```python
from build123d import *

# Parameters (mm, degrees)
SALIENTE_EXTRUIR1_DEPTH = 14
CROQUIS3_R              = 1.75
CORTAR_EXTRUIR1_DEPTH   = 30
REDONDEO3_R             = 4
REDONDEO4_R             = 2


with BuildPart() as part:
    # Croquis2 → Saliente-Extruir1 (new, symmetric)
    with BuildSketch(Plane(origin=(0, 0, 0), x_dir=(0, 0, -1), z_dir=(1, 0, 0))):
        with BuildLine():
            Line((-3, 1.5), (8, 1.5))
            Line((8, 1.5), (8, -1.5))
            Line((8, -1.5), (-8, -1.5))
            Line((-8, -1.5), (-8, 1.5))
            Line((-8, 1.5), (-8, 13.5))
            Line((-8, 13.5), (-5, 13.5))
            Line((-5, 13.5), (-5, 3.5))
            ThreePointArc((-5, 3.5), (-4.414213562, 2.085786438), (-3, 1.5))
        make_face()
    extrude(amount=SALIENTE_EXTRUIR1_DEPTH, both=True)

    # Croquis3 → Cortar-Extruir1 (cut)
    with BuildSketch(Plane(origin=(0, 1.5, 0), x_dir=(1, 0, 0), z_dir=(0, 1, 0))):
        with BuildLine():
            Line((-9, -2), (9, -2))
            Line((9, -2), (9, 1))
            Line((9, 1), (6.5, 1))
            Line((6.5, 1), (6.5, 4.25))
            ThreePointArc((6.5, 4.25), (7.598349575, 6.901650434), (10.250000013, 8))
            Line((10.250000013, 8), (6.5, 8))
            Line((6.5, 8), (-6.5, 8))
            Line((-6.5, 8), (-10.249999997, 8))
            ThreePointArc((-10.249999997, 8), (-7.598349569, 6.901650428), (-6.5, 4.25))
            Line((-6.5, 4.25), (-6.5, 1))
            Line((-6.5, 1), (-9, 1))
            Line((-9, 1), (-9, -2))
        make_face()
        with BuildLine():
            Line((14, 8), (10.250000013, 8))
            ThreePointArc((10.250000013, 8), (12.901650434, 6.901650425), (14, 4.25))
            Line((14, 4.25), (14, 8))
        make_face()
        with BuildLine():
            ThreePointArc((-14, 4.25), (-12.901650428, 6.901650431), (-10.249999997, 8))
            Line((-10.249999997, 8), (-14, 8))
            Line((-14, 8), (-14, 4.25))
        make_face()
        with Locations(Location((9.95, 4, 0), (0, 0, 270))):
            Circle(CROQUIS3_R)
        with Locations(Location((-9.95, 4, 0), (0, 0, 270))):
            Circle(CROQUIS3_R)
    extrude(amount=-CORTAR_EXTRUIR1_DEPTH, mode=Mode.SUBTRACT)

    # Redondeo3
    redondeo3_edges = [part.edges().sort_by_distance(p)[0] for p in [
        (-14, 13.5, 6.5),
        (14, 13.5, 6.5),
    ]]
    fillet(redondeo3_edges, radius=REDONDEO3_R)

    # Redondeo4
    redondeo4_edges = [part.edges().sort_by_distance(p)[0] for p in [
        (6.5, 0, -1),
        (-6.5, 0, -1),
    ]]
    fillet(redondeo4_edges, radius=REDONDEO4_R)


solid = part.part
```
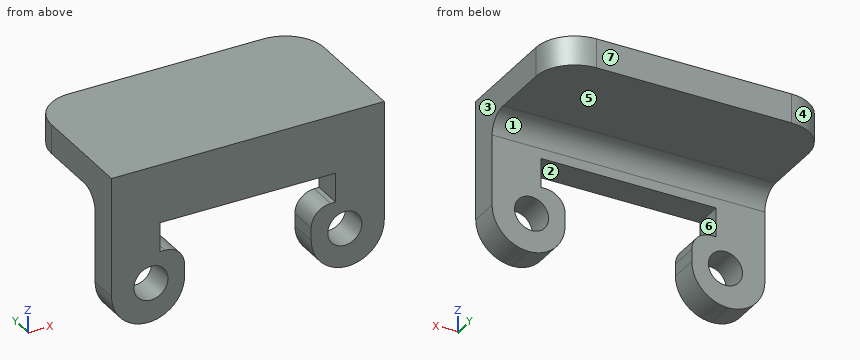
Here's how the part is built. I have some questions about the finished solid (model axes, mm). Face numbers are marked on the shaded views. A direction names the side the tool comes from. Give positions to 0.01 mm unless a question says otherwise; leave off trailing zeros. Loops run counter-clockwise (first coordinate to the right, second up) from the corner with the lowest first, then second, coordinate; pieces in that order, holes last. Notation, with made-up numbers: (19, 76) -> (60, 76) arc R6 cw to (60, 85) -> close; hole circle Ø11 at (71, -26.75). An arc over 180 degrees is marked (long way). Use one line per item in the form item = value. Start each with the question number.
1) Thinking about a two-plate mould opening in X: for the marked faces 1, 2, 3 and 4, which applies, +X half, -X half, draft (parallel to the pull), parting line (faces both ways), or undercut?
2) Imagine slicing it at B-B (x = 0.5). Please give me the cut outline in (y, z), then the cut area to 3 significant figures.
3) Please list where these lines run through material, in increasing order: line 1 along X through (y, z) = (-0.35, -4); line 2 along Y through (x, z) = (-9.5, 1.5); line 3 along Z through (x, y) = (-3.75, 5.75).
4) Imagine slicing it at C-C (z = 6.5). Please give me the cut outline in (x, y).
5) Which directions (+Z, -Z, +X, -X, +Y, -Y) give clear straight access to the entire face, cutting with the end or side of a thin tool? Please do the marked faces 5, 6 and 7.
6) For P1, Ø1, axis at x = -6.5, y = 9, coming from the -Z side; P2, Ø3.5, axis at x = -4, y = -0.5, coming from the -Z side; P3, Ø4, axis at x = 9.95, z = -4, coming from the +Y side, each with a flat end and sliding along its axis, tell me the tip position at first contact or that it passes through.
7) Imagine slicing it at D-D (z = 4.25). Please give me the cut outline in (x, y), then the cut area to 3 significant figures.
8) Imagine slicing it at A-A (z = -0.5). Please give me the cut outline in (x, y).
Check values:
q1.face_1 = draft
q1.face_2 = undercut
q1.face_3 = +X half
q1.face_4 = -X half
q2.outline = (-1.5, 2) -> (1.5, 2) -> (1.5, 3) arc R2 cw to (3.5, 5) -> (13.5, 5) -> (13.5, 8) -> (-1.5, 8) -> close
q2.area = 54.9 mm^2
q3.line_1 = -14 to -11.7, -8.2 to -6.5, 6.5 to 8.2, 11.7 to 14
q3.line_2 = -1.5 to 1.5
q3.line_3 = 5 to 8
q4.outline = (-14, -1.5) -> (14, -1.5) -> (14, 9.5) arc R4 ccw to (10, 13.5) -> (-10, 13.5) arc R4 ccw to (-14, 9.5) -> close
q5.face_5 = -Z, +X, -X, +Y
q5.face_6 = +Y, -Y
q5.face_7 = +Z, -Z, +X, -X, +Y
q6.P1 = 5
q6.P2 = 2
q6.P3 = 1.5
q7.outline = (-14, -1.5) -> (14, -1.5) -> (14, 1.94) -> (-14, 1.94) -> close
q7.area = 96.3 mm^2
q8.outline = (-14, -1.5) -> (-9, -1.5) -> (-9, 1.5) -> (-14, 1.5) -> close; (9, -1.5) -> (14, -1.5) -> (14, 1.5) -> (9, 1.5) -> close
